Build history of the part. All positions in model axes, mm. A direction names the side the tool comes from. Round coordinates to 2 decimals unless told otherwise and drop trailing zeros. Loops run counter-clockwise (first coordinate to the right, second up) from the corner with the lowest first, then second, coordinate; pieces in that order, holes last. Notation, with made-up numbers: (-33.75, 64.25) -> (1.25, 64.25) arc R25 cw to (1.25, 80.25) -> close; hole circle Ø7 at (-32.5, 51). An arc over 180 degrees is marked (long way). Put each result on its own line as item: value. Start each with the question number.
```python
from build123d import *

# Parameters (mm, degrees)
F1_DEPTH = 25.4
F2_W     = 25.9
F2_H     = 25.778546
F3_DEPTH = 4
F4_DEPTH = 25.401


with BuildPart() as f1:
    # F0 (on Front) → F1 (new body)
    with BuildSketch(Plane.XZ):
        Polygon((-47.05, 25.021454), (-88.9, 25.021454), (-88.9, -30.673691), (-88.9, -51.178546), (-41.565981, -51.178546), (0, -51.178546), (88.9, -51.178546), (88.9, 25.021454), (47.05, 25.021454), (47.05, -13.078546), (0, -13.078546), (-47.05, -13.078546), align=None)
    extrude(amount=F1_DEPTH)

    # F2 (on Front) → F3 (cut)
    with BuildSketch(Plane.XZ):
        with Locations((0, -38.289273)):
            Rectangle(F2_W, F2_H)
    extrude(amount=F3_DEPTH, mode=Mode.SUBTRACT)

    # F2 (on Front) → F4 (cut, through all)
    with BuildSketch(Plane.XZ):
        with Locations((0, -38.289273)):
            Rectangle(F2_W, F2_H)
    extrude(amount=F4_DEPTH, mode=Mode.SUBTRACT)


solid = f1.part
```
Item 1: Cut at C-C on z = 9. Write the cut outline in (x, y).
Item 2: Wall check: line 1 (X direction, y = -8, z = -32); line 2 (X direction, y = -19, z = 11); line 3 (Z direction, x = -42, y = -3.75). Give the ranges that are in metal, low to high. Write a range as from..to.
Item 3: Cut at D-D on x = 32.5. Write the cut outline in (y, z).
Item 4: 3-axis set-ups, long thin cutter, end or side, ignore diameter. For faces 5 (the face through (-47.05, -13, 6)), 6 (the face through (0, -13, -25.4)), 7 (the face through (-1, 0, -21)): which of +Z, -Z, +X, -X, +Y, -Y reach the whole face in a straight line?
Item 5: Cut at A-A on z = -41.5. Write the cut outline in (x, y), then the cut area to 3 significant figures.
Item 6: Pull direction X, two halves, no side cores. Call faces 1 (the face through (-1, -25.4, -21)), 2 (the face through (88.9, -13, -14)), 3 (the face through (12.95, -13, -38)), 4 (the face through (-88.9, -13, -13)): +X half, -X half, draft (parallel to the pull), parting line (faces both ways), or undercut.
Item 7: Drop flat-ended pins along their axis: pin 1 (12 mm diameter, centred on x = 7.5, y = -4.5, fed in from +Z); pin 2 (3 mm diameter, centred on x = -0.5, y = -12, fed in from -Z). Give the stop position or say it passes through.
Item 8: Cut at B-B on y = -4.75. Write the cut outline in (x, z).
Ans:
1. outline: (-88.9, -25.4) -> (-47.05, -25.4) -> (-47.05, 0) -> (-88.9, 0) -> close; (47.05, -25.4) -> (88.9, -25.4) -> (88.9, 0) -> (47.05, 0) -> close
2. line 1: x = -88.9..-12.95, 12.95..88.9
2. line 2: x = -88.9..-47.05, 47.05..88.9
2. line 3: z = -51.18..-13.08
3. outline: (-25.4, -51.18) -> (0, -51.18) -> (0, -13.08) -> (-25.4, -13.08) -> close
4. face 5: +Z, +Y, -Y
4. face 6: -Z, +Y, -Y
4. face 7: +Z, -Z, +X, -X, +Y
5. outline: (-88.9, -25.4) -> (-12.95, -25.4) -> (-12.95, 0) -> (-88.9, 0) -> close; (12.95, -25.4) -> (88.9, -25.4) -> (88.9, 0) -> (12.95, 0) -> close
5. area: 3,860 mm2
6. face 1: draft
6. face 2: +X half
6. face 3: undercut
6. face 4: -X half
7. pin 1: stops at z = -13.08
7. pin 2: stops at z = -25.4
8. outline: (-88.9, -51.18) -> (-12.95, -51.18) -> (-12.95, -25.4) -> (12.95, -25.4) -> (12.95, -51.18) -> (88.9, -51.18) -> (88.9, 25.02) -> (47.05, 25.02) -> (47.05, -13.08) -> (-47.05, -13.08) -> (-47.05, 25.02) -> (-88.9, 25.02) -> close
